Verification items for the finished model (mm, model axes). A direction names the side the tool comes from. Give positions to 0.01 mm unless a question says otherwise; leave off trailing zeros. Loops run counter-clockwise (first coordinate to the right, second up) from the corner with the lowest first, then second, coordinate; pieces in that order, holes last. Notation, with made-up numbers: (-23, 31) -> (27, 31) arc R31 cw to (27, 55) -> close; hole circle Ø8 at (77.5, -16). An arc over 180 degrees is marked (long way). Use one line per item in the form item = value. Start each with the question number.
from build123d import *

# Parameters (mm, degrees)
F0_W          = 102.824826
F0_H          = 85.087308
F2_DEPTH      = 175.62094
F3_DEPTH      = 186.03524
F3_DEPTH_BACK = 10.57893
F4_DEPTH      = 63.5


with BuildPart() as f2:
    # F0 (on Front) → F2 (new body)
    with BuildSketch(Plane.XZ):
        with Locations((-13.792595, -34.067582)):
            Rectangle(F0_W, F0_H)
    extrude(amount=F2_DEPTH)

    # F1 (on Front) → F3 (join, two sides)
    with BuildSketch(Plane.XZ) as f3_sk:
        with BuildLine():
            ThreePointArc((50.319818, 8.476072), (18.556965, 37.672102), (-13.180182, 66.896072))
            ThreePointArc((-13.180182, 66.896072), (-45.789547, 37.959676), (-77.905008, 8.476072))
            Line((-77.905008, 8.476072), (50.319818, 8.476072))
        make_face()
    extrude(amount=F3_DEPTH)
    extrude(f3_sk.sketch, amount=-F3_DEPTH_BACK)

    # F0 (on Front) → F4 (join)
    with BuildSketch(Plane.XZ):
        with Locations((-13.792595, -34.067582)):
            Rectangle(F0_W, F0_H)
    extrude(amount=F4_DEPTH)


solid = f2.part
Item 1: Tool access check on faces 1 (the flat face through (-15, -175.621, -33)), 2 (the flat face through (-65.205, -87, -35)), 3 (the flat face through (37.62, -87, -35)). Record the directions out of +Z, -Z, +X, -X, +Y, -Y that give a thin tool (end or side, any length) a straight path to the whole face; none if there is none.
Item 2: Sectioned sample at B-B, the plane x = -6. Enter the section's corners in (y, z), and give its area (3 significant figures).
Item 3: Sectioned sample at D-D, the plane x = -21.5. Enter the section's corners in (y, z).
Item 4: Gauge pin test, flat ends, axial feed: pin 1 Ø8 at (x, z) = (-9.5, -7.5) entering from -Y; pin 2 Ø4 at (x, z) = (36, -14.5) entering from +Y; pin 3 Ø10 at (y, z) = (-145.5, 35.5) entering from -X. Record the tip position at first contact, or that the pin passes through.
Item 5: Sectioned sample at A-A, the plane y = -77. Enter the section's corners in (x, z) (3 decimals), and give its area (3 significant figures).
Item 6: Sectioned sample at C-C, the plane z = -49. Enter the section's corners in (x, y) (3 decimals), and give its area (3 significant figures).
Item 7: Material ranges on line 1 (X direction, y = -172.5, z = -63) (3 decimals); line 2 (Y direction, x = -36.5, z = 1); line 3 (Z direction, x = -71, y = -25), recorded low to high.
Outcome:
q1.face_1 = -Z, +X, -X, -Y
q1.face_2 = -Z, -X, +Y, -Y
q1.face_3 = -Z, +X, +Y, -Y
q2.outline = (-186.04, 8.48) -> (-175.62, 8.48) -> (-175.62, -76.61) -> (0, -76.61) -> (0, 8.48) -> (10.58, 8.48) -> (10.58, 60.28) -> (-186.04, 60.28) -> close
q2.area = 25,100 mm^2
q3.outline = (-186.04, 8.48) -> (-175.62, 8.48) -> (-175.62, -76.61) -> (0, -76.61) -> (0, 8.48) -> (10.58, 8.48) -> (10.58, 59.61) -> (-186.04, 59.61) -> close
q4.pin_1 = -175.62
q4.pin_2 = 0
q4.pin_3 = -54.02
q5.outline = (-77.905, 8.476) -> (-65.205, 8.476) -> (-65.205, -76.611) -> (37.62, -76.611) -> (37.62, 8.476) -> (50.32, 8.476) arc R49024.677 cw to (-13.18, 66.896) arc R2578.454 ccw to start
q5.area = 12,500 mm^2
q6.outline = (-65.205, -175.621) -> (37.62, -175.621) -> (37.62, 0) -> (-65.205, 0) -> close
q6.area = 18,100 mm^2
q7.line_1 = -65.205 to 37.62
q7.line_2 = -175.62 to 0
q7.line_3 = 8.48 to 14.9
